Check sheet for the modelled part. Datum: model origin and axes. Units: mm. Coordinates: 2 decimals unless noted, no trailing zeros. Loops run counter-clockwise (first coordinate to the right, second up) from the corner with the lowest first, then second, coordinate; pieces in that order, holes last. Notation, with made-up numbers: M 0.5,52.5 L 24.5,52.5 A8 ccw 24.5,60.5 Z; hole C -39.5,47 d3. An arc over 180 degrees is marked long. Return JSON: item names as keys, results as strings.
from build123d import *

# Parameters (mm, degrees)
ENL_V_MAT_EXTRU_1_DEPTH      = 7.8
ENL_V_MAT_EXTRU_1_DEPTH_BACK = 7.8
ESQUISSE2_W                  = 52
ESQUISSE2_H                  = 52
ESQUISSE3_R                  = 4.875
BOSS_EXTRU_1_DEPTH           = 3.4


with BuildPart() as part:
    # Esquisse1 → Révolution1 (revolve)
    with BuildSketch(Plane(origin=(0, 0, 0), x_dir=(1, 0, 0), z_dir=(0, 1, 0)), mode=Mode.PRIVATE) as r_volution1_sk:
        Polygon((0, -6.5), (3.4, -19.188972746), (6.8, -6.5), (6.8, -4), (6.1235, -3.3235), (0.6765, -3.3235), (0, -4), align=None)
    revolve(r_volution1_sk.sketch.rotate(Axis((0, 0, 0), (1, 0, 0)), 180), axis=Axis((0, 0, 0), (1, 0, 0)))

    # Esquisse2 → Enlèv. mat.-Extru.1 (cut, two sides: drawn at the far end of the back side and taken through both)
    with BuildSketch(Plane(origin=(0, 0, 0), x_dir=(0, 0, -1), z_dir=(1, 0, 0)).offset(-ENL_V_MAT_EXTRU_1_DEPTH_BACK)):
        Rectangle(ESQUISSE2_W, ESQUISSE2_H)
        Polygon((-6.5, -3.75277675), (0, -7.505553499), (6.5, -3.75277675), (6.5, 3.75277675), (0, 7.505553499), (-6.5, 3.75277675), align=None, mode=Mode.SUBTRACT)
    extrude(amount=ENL_V_MAT_EXTRU_1_DEPTH + ENL_V_MAT_EXTRU_1_DEPTH_BACK, mode=Mode.SUBTRACT)


with BuildPart() as body_2:
    # Esquisse3 → Boss.-Extru.1 (new body)
    with BuildSketch(Plane(origin=(0, 0, 0), x_dir=(0, 0, -1), z_dir=(1, 0, 0))):
        with Locations(Location((0, 0, 0), (0, 0, 180))):
            Circle(ESQUISSE3_R)
    extrude(amount=BOSS_EXTRU_1_DEPTH)

    # SupprimerFace1: 1 face struck out; the rest of the skin is kept as a surface, the solid goes
    supprimerface1_1_drop = [body_2.part.faces().sort_by_distance(Vector(p))[0] for p in ((3.4, 0, 0),)]
    supprimerface1_1 = Shell(body_2.part.faces() - supprimerface1_1_drop)


solid = part.part
1) Draft check along Z on faces 1 (the face through (0.065, 3.358, -5.849)), 2 (the face through (3.36, -2.95, -1.53)), 3 (the face through (0.065, 3.386, 5.833)). Enter one of: +Z half, -Z half, draft (parallel to the pull), parting line (faces both ways), or undercut.
Answers:
{"face 1": "-Z half", "face 2": "undercut", "face 3": "+Z half"}
2) Section check A-A on x = 5.5. Record the cut outline in (y, z).
Answers:
{"outline": "M -7.51,0 L -3.75,-6.5 L 3.75,-6.5 L 7.51,0 L 3.75,6.5 L -3.75,6.5 Z; hole C 0,0 d6.65"}
3) Scan lines: line 1 along Z through (x, y) = (5, -1.5); line 2 along Y through (x, z) = (4.5, -1); line 3 along Z through (x, y) = (2.25, -3). Record each from-to range of solid material in increasing order. Write a range as [from, to].
Answers:
{"line 1": "[-6.5, -2.97], [2.97, 6.5]", "line 2": "[-6.93, -3.17], [3.17, 6.93]", "line 3": "[-6.5, -1.43], [1.43, 6.5]"}
4) Go/stop test with flat-tipped pins: pin 1 Ø2 at (x, z) = (3.5, 3) entering from -Y; pin 2 Ø2 at (y, z) = (2.5, 1.5) entering from -X. Record where each tip stops, or that it passes through.
Answers:
{"pin 1": "y = -6.35", "pin 2": "x = 0.08"}
